Could you check a few things on this model? Use its own coordinates, in mm. Give positions to 0.01 mm unless a question says otherwise; leave off trailing zeros. Order: outer loops, then holes, each group sorted by start corner. A loop starts at its lowest first (then second) coordinate and runs counter-clockwise, first axis right, second up. Notation, with made-up numbers: M 87.5,12.5 L 130.5,12.5 A19 ccw 130.5,47.5 Z; hole C 52,83.5 d10. An arc over 180 degrees is marked long. Return JSON: item names as keys, results as strings. Group by question number.
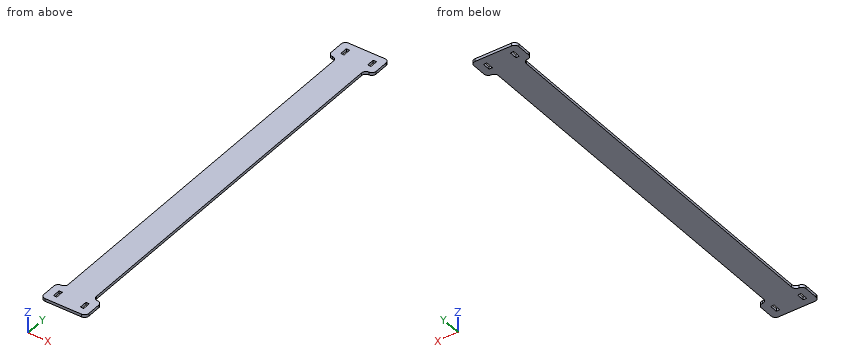
```python
from build123d import *

# Parameters (mm, degrees)
F0_W     = 1.905
F0_H     = 4.445
F1_DEPTH = 1.5875
F2_R     = 2.38124


# Not quite as in the source:
# - a fillet or chamfer is up to 0.001 mm smaller than in the source, because OpenCascade refuses the exact size


with BuildPart() as f1:
    # F0 (on Top) → F1 (new body)
    with BuildSketch(Plane.XY):
        Polygon((-69.85, 120.65), (-95.25, 120.65), (-95.25, 107.95), (-90.4875, 107.95), (-90.4875, -107.95), (-95.25, -107.95), (-95.25, -120.65), (-69.85, -120.65), (-69.85, -107.95), (-74.6125, -107.95), (-74.6125, 107.95), (-69.85, 107.95), align=None)
        with Locations((-90.17, -114.3)):
            Rectangle(F0_W, F0_H, mode=Mode.SUBTRACT)
        with Locations((-74.93, -114.3)):
            Rectangle(F0_W, F0_H, mode=Mode.SUBTRACT)
        with Locations((-90.17, 114.3)):
            Rectangle(F0_W, F0_H, mode=Mode.SUBTRACT)
        with Locations((-74.93, 114.3)):
            Rectangle(F0_W, F0_H, mode=Mode.SUBTRACT)
    extrude(amount=F1_DEPTH)

    # F2 (radius 2.38125 in the source; OpenCascade refuses exactly that, so slightly less here)
    f2_edges = [f1.edges().sort_by_distance(p)[0] for p in [
        (-90.4875, -107.95, 0.79375),
        (-95.25, -107.95, 0.79375),
        (-95.25, -120.65, 0.79375),
        (-69.85, -120.65, 0.79375),
        (-69.85, -107.95, 0.79375),
        (-74.6125, -107.95, 0.79375),
        (-69.85, 120.65, 0.79375),
        (-69.85, 107.95, 0.79375),
        (-95.25, 120.65, 0.79375),
        (-95.25, 107.95, 0.79375),
        (-74.6125, 107.95, 0.79375),
        (-90.4875, 107.95, 0.79375),
    ]]
    fillet(f2_edges, radius=F2_R)


solid = f1.part
```
1. Imagine slicing it at B-B, the plane z = 0.95. Count the separate pieces of the cut face and the enclosed holes in it, plus the area to 3 significant figures.
2. I need wall thicknesses on L1, parallel to Y at x = -75.25, z = 0.85; L2, parallel to X at y = 100, z = 1.4; L3, parallel to Y at x = -91, z = 0.95. Which ranges of each line are inside material? Lowest first, please. Write a range as from..to.
3. Imagine slicing it at A-A, the plane y = -74. Please give me the cut outline in (x, z), plus the area to 3 significant figures.
4. For pin 1 (10 mm diameter, centred on x = -82.5, y = -72.5, fed in from -Z); pin 2 (0.5 mm diameter, centred on y = -23, z = 0.5, fed in from +X), each with a flat end and sliding along its axis, tell me the tip position at first contact or that it passes through.
Values:
{
 "1": {"separate pieces": "1", "enclosed holes": "4", "area": "4,030 mm²"},
 "2": {"L1": "y = -120.65..-116.52, -112.08..112.08, 116.52..120.65", "L2": "x = -90.49..-74.61", "L3": "y = -120.65..-116.52, -112.08..-107.04, 107.04..112.08, 116.52..120.65"},
 "3": {"outline": "M -90.49,0 L -74.61,0 L -74.61,1.59 L -90.49,1.59 Z", "area": "25.2 mm²"},
 "4": {"pin 1": "stops at z = 0", "pin 2": "stops at x = -74.61"}
}
